Check sheet for the modelled part. Datum: model origin and axes. Units: mm. Face numbers are marked on the shaded views. A direction names the side the tool comes from. Round coordinates to 2 decimals unless told otherwise and drop trailing zeros. Write each loop counter-clockwise with the first axis right and the second up, starting at its lowest first coordinate (ties: lowest second). Pieces come first, ordered by that corner, then holes. Notation, with made-up numbers: (35.25, -34.75) -> (72.25, -34.75) arc R21 cw to (72.25, 4.25) -> close; hole circle Ø2 at (72.5, -18). An arc over 180 degrees is marked (long way). One line per item, written item: value.
Autodesk Inventor part; units mm, degrees
ref_plane "YZ Plane" through (0, 0, 0) normal (1, 0, 0) x (0, 1, 0)
ref_plane "XZ Plane" through (0, 0, 0) normal (0, 1, 0) x (-1, 0, 0)
ref_plane "XY Plane" through (0, 0, 0) normal (0, 0, 1) x (1, 0, 0)
sketch "Sketch1" plane through (0, 0, 0) normal (0, 0, 1) x (1, 0, 0)
  circle A0 centre (0, 0) radius 5
  dimension "d0" = 10
extrude "Extrusion1" add sketch "Sketch1" along normal mid plane 40
sketch "Sketch2" plane through (0, 0, 20) normal (0, 0, 1) x (1, 0, 0)
  circle A0 centre (0, 0) radius 4
  line L0 (-2.6458, 3) -> (2.6458, 3)
  line L1 (1.5, 2.5) -> (1.5, 5.5)
  line L2 (1.5, 5.5) -> (-1.5, 5.5)
  line L3 (-1.5, 5.5) -> (-1.5, 2.5)
  line L4 (-1.5, 2.5) -> (1.5, 2.5)
  line L5 (1.5, 2.5) -> (-1.5, 5.5) construction
  line L6 (1.5, 5.5) -> (-1.5, 2.5) construction
  line L7 (0, -7.1) -> (0, 7.6)
  point P0 (0, 4)
  point P1 (0, 4)
  point P2 (-1.5, 3.7081)
  point P3 (1.5, 3.7081)
  dimension "d3" = 8
  dimension "d4" = 3
  dimension "d11" = 3
  dimension "d12" = 3
extrude "Extrusion2" add sketch "Sketch2" along normal blind 16.5 contours A0 L7 L4 L1 L0 | L0 L1 A0 | A0 L0 L3 L4 L7 | L1 L0 L7 A0 | L1 L4 L7 L0 | A0 L3 L0 | L4 L3 L0 L7 | L7 L0 L3 A0
thread "Thread1"
mirror "Mirror2" about plane through (0, 0, 0) normal (0, 0, 1) of "Extrusion2"
thread "Thread2"
extrude "Extrusion3" cut sketch "Sketch2" along normal through all both and the other way through all contours L1 L0 L7 A0 | A0 L7 L2 L1 | L1 L4 L7 L0 | L4 L3 L0 L7 | L7 L0 L3 A0 | A0 L3 L2 L7
properties part number "HornGearShaft" material "Stainless Steel"
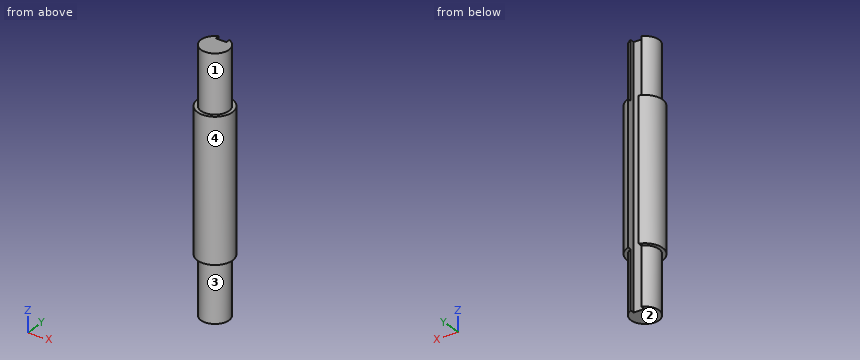
Item 1: Tool access check on the marked faces 3 and 4. Record the directions out of +Z, -Z, +X, -X, +Y, -Y that give a thin tool (end or side, any length) a straight path to the whole face; none if there is none.
Answer:
face 3: -Z
face 4: +Z, -Z
Item 2: Depth check by flat-ended pin: P1, Ø5, axis at y = 3.5, z = 18, coming from the +X side; P2, Ø0.9, axis at x = 0, z = -16.5, coming from the +Y side; P3, Ø3, axis at y = 0, z = -22.5, coming from the +X side. Enter the tip coordinate at first touch or a pass-through.
Answer:
P1: stops at x = 4.9
P2: stops at y = 2.5
P3: stops at x = 4
Item 3: Mould release check, pull along X, two halves, no side actions. Record for the marked faces 1 and 2: pulls with the +X half, pulls with the -X half, needs draft (parallel to the pull), parting line crosses it, or undercut.
Answer:
face 1: parting line crosses it
face 2: needs draft
Item 4: Sectioned sample at A-A on x = 0. Enter the section's corners in (y, z).
Answer:
outline: (-5, -20) -> (-4, -20) -> (-4, -36.5) -> (2.5, -36.5) -> (2.5, 36.5) -> (-4, 36.5) -> (-4, 20) -> (-5, 20) -> close
Item 5: Sectioned sample at D-D on z = 9. Enter the section's corners in (x, y).
Answer:
outline: (-1.5, 2.5) -> (-1.5, 4.77) arc R5 ccw (long way) to (1.5, 4.77) -> (1.5, 2.5) -> close
Item 6: Sectioned sample at B-B on y = 0. Enter the section's corners in (x, z), and give its area (3 significant figures).
Answer:
outline: (-5, -20) -> (-4, -20) -> (-4, -36.5) -> (4, -36.5) -> (4, -20) -> (5, -20) -> (5, 20) -> (4, 20) -> (4, 36.5) -> (-4, 36.5) -> (-4, 20) -> (-5, 20) -> close
area: 664 mm^2
Item 7: Sectioned sample at C-C on z = -21.5. Enter the section's corners in (x, y).
Answer:
outline: (-1.5, 2.5) -> (-1.5, 3.71) arc R4 ccw (long way) to (1.5, 3.71) -> (1.5, 2.5) -> close
Item 8: Thickness scan on line 1 (Z direction, x = 4, y = -1.5); line 2 (X direction, y = 3.5, z = -22.5); line 3 (X direction, y = 2.75, z = 33.5). Record the ranges inside material, lowest first.
Answer:
line 1: z = -20 to 20
line 2: x = -1.94 to -1.5, 1.5 to 1.94
line 3: x = -2.9 to -1.5, 1.5 to 2.9
